Read the model definition and answer for the solid it produces. Units are mm, in the model's axes. A direction names the side the tool comes from. Coordinates: 2 decimals unless noted, no trailing zeros. Loops run counter-clockwise (first coordinate to the right, second up) from the corner with the lowest first, then second, coordinate; pieces in that order, holes last. Notation, with made-up numbers: (-8, 4) - (45, 4) arc R31 ccw to (45, 36) - close; hole circle Ø8 at (4, -10). An arc over 180 degrees is marked (long way). Use CSV: the item, a comma, the result in double quotes.
```python
from build123d import *

# Parameters (mm, degrees)
F0_R     = 23.2102979376
F1_DEPTH = 25


with BuildPart() as f1:
    # F0 (on Top) → F1 (new body)
    with BuildSketch(Plane.XY):
        with Locations((-52.1805621684, 40.0566533208)):
            Circle(F0_R)
        with BuildLine():
            ThreePointArc((-35.2217002906, 46.6907966038), (-34.2858599457, 43.4322252204), (-33.970266913, 40.0566533208))
            ThreePointArc((-33.970266913, 40.0566533208), (-34.9955095005, 34.0326332268), (-37.9557946141, 28.6869197569))
            ThreePointArc((-37.9557946141, 28.6869197569), (-45.5464188854, 23.097791443), (-54.9146564918, 22.0527764739))
            ThreePointArc((-54.9146564918, 22.0527764739), (-63.5502957323, 25.8318857665), (-69.1394240461, 33.4225100378))
            ThreePointArc((-69.1394240461, 33.4225100378), (-70.1844390153, 42.7907476443), (-66.4053297227, 51.4263868847))
            ThreePointArc((-66.4053297227, 51.4263868847), (-58.8147054513, 57.0155151985), (-49.4464678449, 58.0605301677))
            ThreePointArc((-49.4464678449, 58.0605301677), (-40.8108286044, 54.2814208751), (-35.2217002906, 46.6907966038))
        make_face(mode=Mode.SUBTRACT)
        with BuildLine():
            Line((-49.4464678449, 58.0605301677), (-35.2217002906, 46.6907966038))
            ThreePointArc((-35.2217002906, 46.6907966038), (-40.8108286044, 54.2814208751), (-49.4464678449, 58.0605301677))
        make_face()
        with BuildLine():
            Line((-66.4053297227, 51.4263868847), (-49.4464678449, 58.0605301677))
            ThreePointArc((-49.4464678449, 58.0605301677), (-58.8147054513, 57.0155151985), (-66.4053297227, 51.4263868847))
        make_face()
        with BuildLine():
            ThreePointArc((-37.9557946141, 28.6869197569), (-34.9955095005, 34.0326332268), (-33.970266913, 40.0566533208))
            ThreePointArc((-33.970266913, 40.0566533208), (-34.2858599457, 43.4322252204), (-35.2217002906, 46.6907966038))
            Line((-35.2217002906, 46.6907966038), (-37.9557946141, 28.6869197569))
        make_face()
        with BuildLine():
            ThreePointArc((-54.9146564918, 22.0527764739), (-45.5464188854, 23.097791443), (-37.9557946141, 28.6869197569))
            Line((-37.9557946141, 28.6869197569), (-54.9146564918, 22.0527764739))
        make_face()
        with BuildLine():
            Line((-69.1394240461, 33.4225100378), (-66.4053297227, 51.4263868847))
            ThreePointArc((-66.4053297227, 51.4263868847), (-70.1844390153, 42.7907476443), (-69.1394240461, 33.4225100378))
        make_face()
        with BuildLine():
            ThreePointArc((-69.1394240461, 33.4225100378), (-63.5502957323, 25.8318857665), (-54.9146564918, 22.0527764739))
            Line((-54.9146564918, 22.0527764739), (-69.1394240461, 33.4225100378))
        make_face()
    extrude(amount=F1_DEPTH)


solid = f1.part
```
Q1. The part is cut by section B-B on x = -64.5. Determine the outline of the cut face in (y, z).
Reported:
outline,"(20.39, 0) - (29.71, 0) - (29.71, 25) - (20.39, 25) - close; (52.17, 0) - (59.73, 0) - (59.73, 25) - (52.17, 25) - close"
Q2. For a pull along X with two mould halves and no side action, classify faces 3 (the face through (-57.212, 17.398, 12.325)), 4 (the face through (-42.434, 52.455, 12.325)), 5 (the face through (-42, 25, 0)) as +X half, -X half, draft (parallel to the pull), parting line (faces both ways), or undercut.
Reported:
face 3,"parting line"
face 4,"undercut"
face 5,"draft"
Q3. Given P1, Ø5, axis at x = -48, z = 13.5, coming from the +Y side; P2, Ø12, axis at y = 25, z = 8, coming from the -X side; P3, Ø2, axis at y = 22.5, z = 20, coming from the +X side, each flat-ended and moving along its own axis, determine where each tip first touches the part or whether it passes through.
Reported:
P1,"stops at y = 63.21"
P2,"stops at x = -73.55"
P3,"stops at x = -35.91"
Q4. A tool of negligible diameter and unlimited length cuts with its end or side. For faces 1 (the face through (-42, 25, 25)), 2 (the face through (-46.317, 25.416, 12.325)), from which of +Z, -Z, +X, -X, +Y, -Y can it reach the whole face along a straight path? Write none if from no direction.
Reported:
face 1,"+Z, +X, -X, +Y, -Y"
face 2,"+Z, -Z"
Q5. The part is cut by section D-D on x = -71.5. Determine the outline of the cut face in (y, z).
Reported:
outline,"(27.19, 0) - (52.92, 0) - (52.92, 25) - (27.19, 25) - close"
Q6. Find the intervals of material crossed by probe 1 along Y at (x, z) = (-56.5, 9.25); probe 2 along Y at (x, z) = (-57, 10.75); probe 3 along X at (y, z) = (42, 11.5), in increasing order. Write a range as [from, to].
Reported:
probe 1,"y = [17.25, 23.32], [55.3, 62.86]"
probe 2,"y = [17.35, 23.72], [55.11, 62.76]"
probe 3,"x = [-75.31, -67.84], [-35.93, -29.05]"
Q7. The part is cut by section A-A on y = 34. Determine the outline of the cut face in (x, z), and give its area (3 significant figures).
Reported:
outline,"(-74.59, 0) - (-69.05, 0) - (-69.05, 25) - (-74.59, 25) - close; (-37.15, 0) - (-29.77, 0) - (-29.77, 25) - (-37.15, 25) - close"
area,"323 mm²"
Q8. The part is cut by section C-C on z = 10.75. Determine the outline of the cut face in (x, y), and give its area (3 significant figures).
Reported:
outline,"circle Ø46.42 at (-52.18, 40.06); hole (-69.14, 33.42) - (-54.91, 22.05) - (-37.96, 28.69) - (-35.22, 46.69) - (-49.45, 58.06) - (-66.41, 51.43) - close"
area,"831 mm²"
